The model under review builds one solid part; all positions refer to its coordinate system, in mm. A direction names the side the tool comes from. Round coordinates to 2 decimals unless told otherwise and drop trailing zeros. Loops run counter-clockwise (first coordinate to the right, second up) from the corner with the lowest first, then second, coordinate; pieces in that order, holes last. Notation, with made-up numbers: M 44.5,88 L 95.5,88 A18 ccw 95.5,107 Z; hole C 32.5,-4 d6. An arc over 180 degrees is marked long. Answer as a JSON object with one key per item and string values. Group by question number.
Item 1: Insertion check: P1, Ø4, axis at x = 5.51, y = -9.52, coming from the +Z side; P2, Ø21.5, axis at x = 5, y = -10, coming from the -Z side; P3, Ø4, axis at y = -31.5, z = 4.5, coming from the -X side; P4, Ø2, axis at x = 22.5, z = 0.5, coming from the +Y side. Each pin has a flat end and moves straight along its axis. Give the tip position at first contact, or say it passes through.
Item 2: To check wall thickness, follow line 1 (Z direction, x = 7, y = -37.5); line 2 (Z direction, x = 1, y = -7); line 3 (X direction, y = 0, z = 1). State the ranges of each line that lie inside material, in increasing order.
Item 3: Consider section B-B (z = 3.75). State how many separate pieces and enclosed holes the cut face has, and give its area (3 significant figures).
Item 4: Consider section D-D (y = -32). Give the boundary of the cut face in (x, z), and give its area (3 significant figures).
Item 5: Consider section C-C (z = -6.75). Give the boundary of the cut face in (x, y).
Item 6: The part is to be moulded in two halves that separate along Z. For faces 4 (the face through (19, -33, -8.8)), 5 (the face through (25.864, -27.911, -3.135)), 6 (the face through (7.624, 11.742, 2.958)), say which applies: +Z half, -Z half, draft (parallel to the pull), parting line (faces both ways), or undercut.
Item 7: Tool access review of faces 1 (the face through (-6.87, 1.49, 2.96)), 2 (the face through (2.13, 6.7, 2.96)), 3 (the face through (7, -11, 0)): name each direction out of +Z, -Z, +X, -X, +Y, -Y from which nothing blocks a thin tool from reaching the whole face with its end or side.
Item 8: Consider section A-A (y = 0). Give the boundary of the cut face in (x, z).
Autodesk Inventor part; units mm, degrees
ref_plane "YZ Plane" through (0, 0, 0) normal (1, 0, 0) x (0, 1, 0)
ref_plane "XZ Plane" through (0, 0, 0) normal (0, 1, 0) x (-1, 0, 0)
ref_plane "XY Plane" through (0, 0, 0) normal (0, 0, 1) x (1, 0, 0)
sketch "스케치2" plane through (0, 0, 0) normal (0, 0, 1) x (1, 0, 0)
  circle A0 centre (0, 0) radius 14
  arc A1 (-12.8234, 5.618) -> (-12.1163, -7.014) centre (0, 0) ccw
  line L0 (-12.1163, -7.014) -> (7.824, -41.4595)
  line L1 (7.824, -41.4595) -> (32.0565, -27.4315)
  line L2 (32.0565, -27.4315) -> (12.1163, 7.014)
  arc A2 (12.1163, 7.014) -> (1.5142, 13.9179) centre (0, 0) ccw
  circle A3 centre (9.5199, 5.511) radius 1.25
  circle A4 centre (-9.5199, -5.511) radius 1.25
  circle A5 centre (-10.6285, 2.8347) radius 1.25
  circle A6 centre (28.2072, -26.7702) radius 1.35
  circle A7 centre (9.1674, -37.7922) radius 1.35
  circle A8 centre (2.8347, 10.6285) radius 1.25
  circle A9 centre (-2.8347, -10.6285) radius 1.25
  circle A10 centre (5.511, -9.5199) radius 1.25
  circle A11 centre (10.6285, -2.8347) radius 1.25
  circle A12 centre (0, 0) radius 7.25
  line L3 (-9.5199, -5.511) -> (9.5199, 5.511)
  line L4 (9.5199, 5.511) -> (-6.2745, -3.6323)
  arc A13 (-11.0126, 8.6443) -> (1.6585, 13.9014) centre (0, 0) ccw
  line L5 (3.9327, -21.2645) -> (16.4817, -14)
  circle A14 centre (9.5199, 5.511) radius 1.25
  circle A15 centre (-9.5199, -5.511) radius 1.25
  circle A16 centre (-10.6285, 2.8347) radius 1.25
  circle A17 centre (-5.511, 9.5199) radius 1.25
  circle A18 centre (2.8347, 10.6285) radius 1.25
  circle A19 centre (0, 0) radius 7.25
  line L6 (-16.4817, 14) -> (-3.9327, 21.2645)
  circle A20 centre (0, 0) radius 5.2
  line L7 (-4.5003, -2.6052) -> (-9.3099, 5.7031)
  line L8 (4.5003, 2.6052) -> (-0.3093, 10.9135)
  arc A21 (13.8078, -2.3119) -> (-2.0119, 13.8547) centre (0, 0) ccw
  arc A22 (-12.881, 5.4846) -> (-4.8714, -13.1251) centre (0, 0) ccw
  arc A23 (-9.3099, 5.7031) -> (-12.881, 5.4846) centre (-11.0408, 4.7011) ccw
  arc A24 (1.6585, 13.9014) -> (-0.3093, 10.9135) centre (1.4216, 11.9155) ccw
  line L9 (17.8441, -36.8125) -> (14.8381, -31.6198)
  line L10 (5.3181, -37.1308) -> (14.8381, -31.6198)
  line L11 (8.3241, -42.3235) -> (5.3181, -37.1308)
  line L12 (17.8441, -36.8125) -> (8.3241, -42.3235)
  circle A25 centre (9.1674, -37.7922) radius 1.35
  line L13 (20.0307, -28.6138) -> (23.0367, -33.8065)
  line L14 (32.5567, -28.2955) -> (23.0367, -33.8065)
  line L15 (29.5507, -23.1028) -> (32.5567, -28.2955)
  line L16 (20.0307, -28.6138) -> (29.5507, -23.1028)
  circle A26 centre (28.2072, -26.7702) radius 1.35
  line L17 (8.3606, -42.1868) -> (5.4548, -37.1673)
  line L18 (5.4548, -37.1673) -> (14.8016, -31.7564)
  line L19 (14.8016, -31.7564) -> (17.7074, -36.776)
  line L20 (17.7074, -36.776) -> (8.3606, -42.1868)
  line L21 (8.3606, -42.1868) -> (8.274, -42.2369)
  line L22 (8.274, -42.2369) -> (32.5066, -28.2089)
  point P0 (0, 0)
  point P1 (6.2745, 3.6323)
  point P2 (-0.2742, -13.9973)
  point P3 (12.2747, -6.7328)
  point P4 (0, 0)
  point P5 (0, 0)
  point P6 (-12.2747, 6.7328)
  point P7 (0.2742, 13.9973)
  point P8 (-12.881, 5.4846)
  point P9 (1.6585, 13.9014)
  dimension "d16" = 2
  dimension "d17" = 0.1
extrude "돌출1" add sketch "스케치2" along normal blind 6 contours A0 A23 L7 A12 L8 A24 | A0 L2 L16 L13 L1 L9 L10 L0 | L2 L1 L13 L16 | A12 L3 L8 | L10 L9 L1 L19 L18 L17 L0 | A12 L3 A20 | L7 L3 A12 | L1 L17 L18 L19 picked at (1.2989, -11.4658)
sketch "스케치8" plane through (0, 0, 0) normal (0, 0, -1) x (-1, 0, 0)
  circle A0 centre (9.5199, -5.511) radius 1.25
  circle A1 centre (2.8347, -10.6285) radius 1.25
  circle A2 centre (-5.511, -9.5199) radius 1.25
  circle A3 centre (-10.6285, -2.8347) radius 1.25
  circle A4 centre (-9.5199, 5.511) radius 1.25
  circle A5 centre (-28.2072, -26.7702) radius 1.35
  circle A6 centre (-9.1674, -37.7922) radius 1.35
  line L0 (-7.824, -41.4595) -> (-32.0565, -27.4315)
  line L1 (12.1163, -7.014) -> (-7.824, -41.4595)
  arc A7 (12.1163, -7.014) -> (12.881, 5.4846) centre (0, 0) ccw
  arc A8 (12.881, 5.4846) -> (9.3099, 5.7031) centre (11.0408, 4.7011) ccw
  line L2 (4.5003, -2.6052) -> (9.3099, 5.7031)
  arc A9 (-4.5003, 2.6052) -> (4.5003, -2.6052) centre (0, 0) ccw
  line L3 (0.3093, 10.9135) -> (-4.5003, 2.6052)
  arc A10 (0.3093, 10.9135) -> (-1.6585, 13.9014) centre (-1.4216, 11.9155) ccw
  arc A11 (-1.6585, 13.9014) -> (-12.1163, 7.014) centre (0, 0) ccw
  line L4 (-32.0565, -27.4315) -> (-12.1163, 7.014)
  line L5 (-32.0565, -27.4315) -> (-7.824, -41.4595)
  line L6 (-34.4039, -32.4845) -> (-32.673, -33.4865)
  arc A12 (-32.673, -33.4865) -> (-29.5985, -32.6665) centre (-31.5458, -31.5392) ccw
  line L7 (-29.5985, -32.6665) -> (-28.5965, -30.9356)
  arc A13 (-27.2301, -30.5712) -> (-28.5965, -30.9356) centre (-27.7311, -31.4366) ccw
  line L8 (-27.2301, -30.5712) -> (-12.9502, -38.8377)
  arc A14 (-12.5858, -40.2041) -> (-12.9502, -38.8377) centre (-13.4512, -39.7031) ccw
  line L9 (-12.5858, -40.2041) -> (-13.5878, -41.935)
  arc A15 (-13.5878, -41.935) -> (-12.7678, -45.0095) centre (-11.6405, -43.0623) ccw
  line L10 (-12.7678, -45.0095) -> (-11.0369, -46.0115)
  arc A16 (-10.6724, -47.378) -> (-11.0369, -46.0115) centre (-11.5379, -46.877) ccw
  line L11 (-10.6724, -47.378) -> (-34.2195, -88.054)
  arc A17 (-35.5859, -88.4184) -> (-34.2195, -88.054) centre (-35.0849, -87.553) ccw
  line L12 (-35.5859, -88.4184) -> (-37.3168, -87.4164)
  arc A18 (-37.3168, -87.4164) -> (-40.3913, -88.2364) centre (-38.444, -89.3637) ccw
  line L13 (-40.3913, -88.2364) -> (-41.8943, -90.8328)
  line L14 (-36.918, -93.7135) -> (-41.8943, -90.8328)
  line L15 (-29.4982, -91.0759) -> (-36.918, -93.7135)
  line L16 (-2.8951, -45.1207) -> (-29.4982, -91.0759)
  line L17 (-4.3028, -37.3729) -> (-2.8951, -45.1207)
  line L18 (-30.2662, -22.3429) -> (-4.3028, -37.3729)
  line L19 (-37.686, -24.9805) -> (-30.2662, -22.3429)
  line L20 (-64.2892, -70.9357) -> (-37.686, -24.9805)
  line L21 (-62.8814, -78.6835) -> (-64.2892, -70.9357)
  line L22 (-57.9051, -81.5642) -> (-62.8814, -78.6835)
  line L23 (-57.9051, -81.5642) -> (-56.4021, -78.9679)
  arc A19 (-56.4021, -78.9679) -> (-57.2221, -75.8934) centre (-58.3493, -77.8406) ccw
  line L24 (-57.2221, -75.8934) -> (-58.953, -74.8914)
  arc A20 (-59.3174, -73.5249) -> (-58.953, -74.8914) centre (-58.452, -74.0259) ccw
  line L25 (-59.3174, -73.5249) -> (-35.7704, -32.8489)
  arc A21 (-34.4039, -32.4845) -> (-35.7704, -32.8489) centre (-34.9049, -33.3499) ccw
  circle A22 centre (-59.6114, -68.444) radius 1.35
  circle A23 centre (-48.5894, -49.4042) radius 1.35
  circle A24 centre (-28.2072, -26.7702) radius 1.35
  circle A25 centre (-29.667, -85.7786) radius 1.35
  circle A26 centre (-18.6449, -66.7388) radius 1.35
  circle A27 centre (-9.1674, -37.7922) radius 1.35
  circle A28 centre (-37.5674, -30.3643) radius 1.35
  circle A29 centre (-7.6229, -47.699) radius 1.35
  point P0 (0, 0)
  point P1 (-29.4008, -22.8439)
  point P2 (-17.2574, -35.9986)
  point P3 (-5.1683, -36.8719)
extrude "돌출4" add sketch "스케치8" along normal blind 8.8 contours L0 L4 L18 L1
sketch "스케치9" plane through (29.4008, -22.8439, 0) normal (-0.5010009, 0.8654468, 0) x (0.8654468, 0.5010009, 0)
  line L0 (-26.35, 8.8) -> (-23.65, 8.8)
  line L1 (-23.65, -6) -> (-26.35, -6)
  line L2 (-25, 8.8) -> (-25, -6)
  line L3 (-25, -2.5) -> (-25, 8.8)
  line L4 (-25, 8.8) -> (-25, -2.5)
  line L5 (-25, 3.15) -> (-27.6, 3.15)
  line L6 (-25, 3.15) -> (-22.4, 3.15)
  line L7 (-22.4, 3.15) -> (-22.4, 2.05)
  line L8 (-22.4, 3.15) -> (-22.4, 4.25)
  line L9 (-22.4, 4.25) -> (-27.6, 4.25)
  line L10 (-27.6, 4.25) -> (-27.6, 2.05)
  line L11 (-27.6, 2.05) -> (-22.4, 2.05)
  line L12 (-22.4, 2.05) -> (-22.4, 4.25)
  line L13 (-28, 0) -> (-28, 8.8)
  line L14 (-27.6, 4.25) -> (-28, 4.25)
  line L15 (-28, 4.25) -> (-28, 2.05)
  line L16 (-28, 2.05) -> (-27.6, 2.05)
  line L17 (-27.6, 2.05) -> (-27.6, 4.25)
  line L18 (0, 0) -> (-28, 0)
  line L19 (-26.35, -6) -> (-26.35, 8.8)
  line L20 (-14, 0) -> (-14, 8.8)
  line L21 (-28, 8.8) -> (0, 8.8)
  line L22 (-3, 3.15) -> (-0.4, 3.15)
  line L23 (-3, 3.15) -> (-5.6, 3.15)
  line L24 (-5.6, 3.15) -> (-5.6, 2.05)
  line L25 (-5.6, 3.15) -> (-5.6, 4.25)
  line L26 (-5.6, 4.25) -> (-0.4, 4.25)
  line L27 (-0.4, 4.25) -> (-0.4, 2.05)
  line L28 (-0.4, 2.05) -> (-5.6, 2.05)
  line L29 (-5.6, 2.05) -> (-5.6, 4.25)
  line L30 (-0.4, 4.25) -> (0, 4.25)
  line L31 (0, 4.25) -> (0, 2.05)
  line L32 (0, 2.05) -> (-0.4, 2.05)
  line L33 (-0.4, 2.05) -> (-0.4, 4.25)
  point P0 (-5.6, 2.05)
  point P1 (-0.4, 2.05)
  dimension "d20" = 2.6
  dimension "d21" = 2.6
  dimension "d22" = 1.1
  dimension "d23" = 1.1
extrude "돌출5" cut sketch "스케치9" against normal up to next contours L19 L5 L10 L9 | L9 L2 L5 L19 | L9 L8 L6 L2 | L10 L16 L13 L14 | L19 L11 L10 L5 | L5 L2 L11 L19 | L6 L7 L11 L2 | L23 L25 L26 L27 L22 | L22 L27 L28 L24 L23 | L27 L30 L31 L32
properties part number "부품47" material "PMMA 플라스틱"
Geometry results:
{
 "1": {"P1": "stops at z = 6", "P2": "stops at z = 0", "P3": "stops at x = 0.9", "P4": "stops at y = -9.2"},
 "2": {"line 1": "z = -8.8 to -4.25, -2.05 to 6", "line 2": "z = 0 to 6", "line 3": "x = -14 to -6.01, 5.2 to 16.18"},
 "3": {"separate pieces": "1", "enclosed holes": "9", "area": "1,190 mm^2"},
 "4": {"outline": "M 2.35,0 L 13.58,0 L 13.58,-8.8 L 24.16,-8.8 L 24.16,6 L 2.35,6 Z", "area": "224 mm^2"},
 "5": {"outline": "M 5.17,-36.87 L 7.82,-41.46 L 32.06,-27.43 L 29.4,-22.84 Z; hole C 9.17,-37.79 d2.7; hole C 28.21,-26.77 d2.7"},
 "6": {"face 4": "-Z half", "face 5": "undercut", "face 6": "draft"},
 "7": {"face 1": "+Z, -Z, +Y", "face 2": "+Z, -Z", "face 3": "-Z, -X, +Y"},
 "8": {"outline": "M -14,0 L -6.01,0 L -6.01,6 L -14,6 Z; M 5.2,0 L 16.18,0 L 16.18,6 L 5.2,6 Z"}
}
